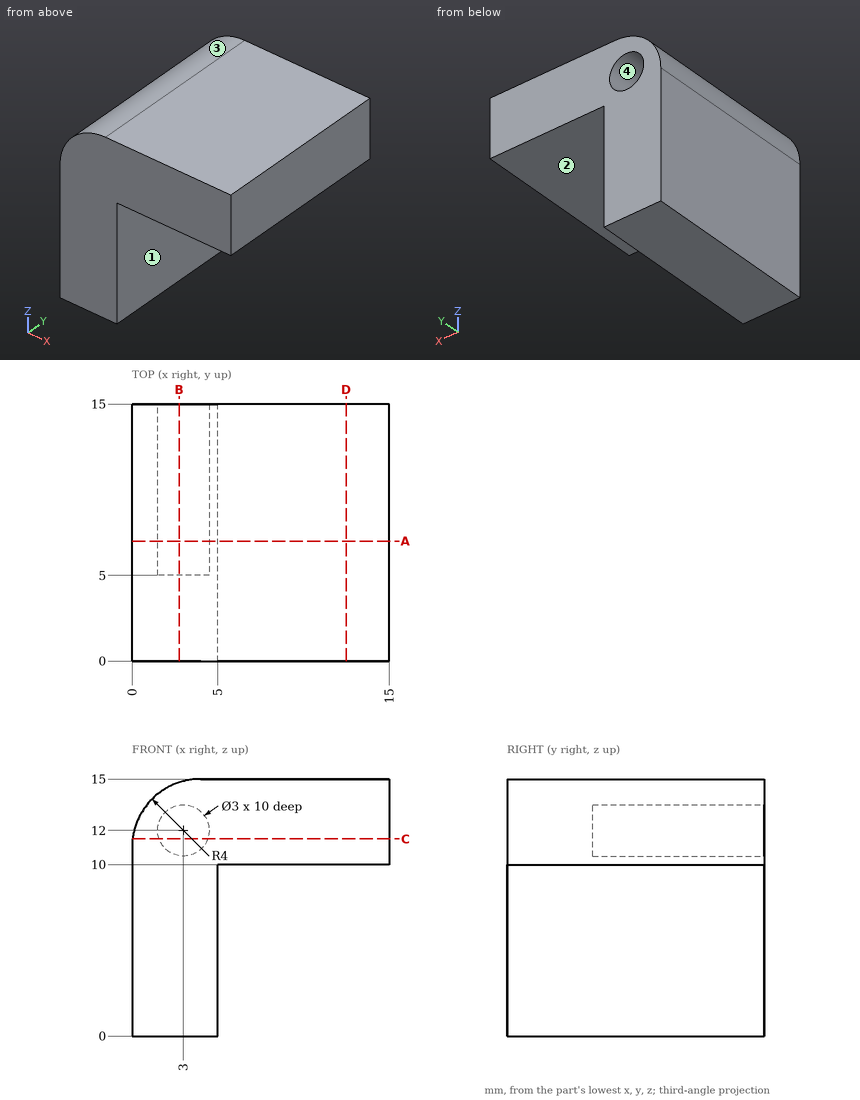
Check sheet for the drawn part. Datum: minimum x, y, z corner. Units: mm. Round coordinates to 2 decimals unless told otherwise and drop trailing zeros. Order: outer loops, then holes, each group sorted by start corner. A loop starts at its lowest first (then second) coordinate and runs counter-clockwise, first axis right, second up. Notation, with made-up numbers: (-3.75, 71) -> (45.25, 71) arc R16 ccw to (45.25, 80) -> close; hole circle Ø3 at (-32, 19.25). An arc over 180 degrees is marked (long way). Put each result on its own line as item: value. Start each with the question number.
(1) Section check B-B (x = 2.75). Enter the section's corners in (y, z), then the cut area to 3 significant figures.
(2) Section check A-A (y = 7). Enter the section's corners in (x, z), then the cut area to 3 significant figures.
(3) Draft check along Z on the marked faces 1, 2, 3 and 4. Enter one of: +Z half, -Z half, draft (parallel to the pull), parting line (faces both ways), or undercut.
(4) Section check C-C (z = 11.5). Enter the section's corners in (x, y), then the cut area to 3 significant figures.
(5) Section check D-D (x = 12.5). Enter the section's corners in (y, z).
(6) Material ranges on line 1 along Z through (x, y) = (3, 9.25); line 2 along X through (y, z) = (7.75, 12); line 3 along Y through (x, z) = (3, 12.5), recorded low to high.
(7) Depth check by flat-ended pin: pin 1 Ø2 at (y, z) = (4, 10.5) entering from -X; pin 2 Ø3 at (y, z) = (9.5, 5) entering from +X; pin 3 Ø3 at (x, y) = (10, 5) entering from -Z. Enter the tip coordinate at first touch or a pass-through.
Completed:
1. outline: (0, 0) -> (15, 0) -> (15, 10.52) -> (5, 10.52) -> (5, 13.48) -> (15, 13.48) -> (15, 14.8) -> (0, 14.8) -> close
1. area: 192 mm2
2. outline: (0, 0) -> (5, 0) -> (5, 10) -> (15, 10) -> (15, 15) -> (4, 15) arc R4 ccw to (0, 11) -> close; hole circle Ø3 at (3, 12)
2. area: 114 mm2
3. face 1: draft
3. face 2: -Z half
3. face 3: +Z half
3. face 4: undercut
4. outline: (0.03, 0) -> (15, 0) -> (15, 15) -> (4.41, 15) -> (4.41, 5) -> (1.59, 5) -> (1.59, 15) -> (0.03, 15) -> close
4. area: 196 mm2
5. outline: (0, 10) -> (15, 10) -> (15, 15) -> (0, 15) -> close
6. line 1: z = 0 to 10.5, 13.5 to 14.87
6. line 2: x = 0.13 to 1.5, 4.5 to 15
6. line 3: y = 0 to 5
7. pin 1: stops at x = 0
7. pin 2: stops at x = 5
7. pin 3: stops at z = 10
